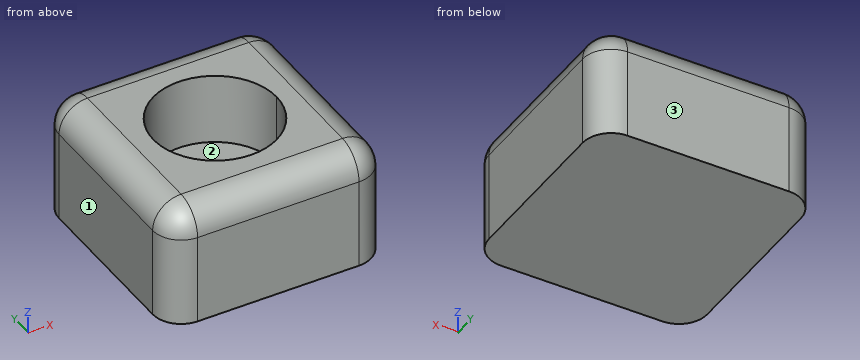
```python
from build123d import *

# Parameters (mm, degrees)
F0_W         = 46
F0_H         = 46
F1_DEPTH     = 25
F3_DEPTH     = 15
F4_R         = 6
F5_T1_DEPTH  = 34
F5_S5_W      = 6
F5_S5_H      = 6
F5_T6_DEPTH  = 6
F5_S11_W     = 6
F5_S11_H     = 6
F5_T12_DEPTH = 6
F5_S17_W     = 6
F5_S17_H     = 6
F5_T18_DEPTH = 6
F5_S23_W     = 6
F5_S23_H     = 6
F5_T24_DEPTH = 6


# Not quite as in the source:
# - a fillet or chamfer that OpenCascade refuses, or shapes differently, is made with other operations: its cross-section is extruded or revolved along the edge and cut away or added


with BuildPart() as f1:
    # F0 (on Top) → F1 (new body)
    with BuildSketch(Plane.XY):
        with Locations((-23, 23)):
            Rectangle(F0_W, F0_H)
    extrude(amount=F1_DEPTH)

    # F2 (on face) → F3 (cut)
    with BuildSketch(Plane.XY.offset(25)):
        with BuildLine():
            ThreePointArc((-10, 23), (-32.1923881554, 32.1923881554), (-23, 10))
            ThreePointArc((-23, 10), (-13.8076118446, 13.8076118446), (-10, 23))
        make_face()
    extrude(amount=-F3_DEPTH, mode=Mode.SUBTRACT)

    # F4
    f4_edges = [f1.edges().sort_by_distance(p)[0] for p in [
        (-23, 0, 25),
        (-46, 23, 25),
        (0, 23, 25),
        (-23, 46, 25),
    ]]
    fillet(f4_edges, radius=F4_R)

    # F5: fillet of radius 6 on 4 edges, made by hand

    # F5_s2 → F5_t1 (cut)
    with BuildSketch(Plane.XY.offset(-15)):
        with BuildLine():
            ThreePointArc((-40, 0), (-44.2426406871, 1.7573593129), (-46, 6))
            Line((-46, 6), (-46, 0))
            Line((-46, 0), (-40, 0))
        make_face()
        with BuildLine():
            ThreePointArc((-6, 0), (-1.7573593129, 1.7573593129), (0, 6))
            Line((0, 6), (0, 0))
            Line((0, 0), (-6, 0))
        make_face()
        with BuildLine():
            ThreePointArc((0, 40), (-1.7573593129, 44.2426406871), (-6, 46))
            Line((-6, 46), (0, 46))
            Line((0, 46), (0, 40))
        make_face()
        with BuildLine():
            ThreePointArc((-46, 40), (-44.2426406871, 44.2426406871), (-40, 46))
            Line((-40, 46), (-46, 46))
            Line((-46, 46), (-46, 40))
        make_face()
    extrude(amount=F5_T1_DEPTH, mode=Mode.SUBTRACT)


with BuildPart() as f5_tool4:
    # F5_s5 → F5_t6 (new body)
    with BuildSketch(Plane.YZ.offset(-40)):
        with Locations((43, 22)):
            Rectangle(F5_S5_W, F5_S5_H)
    extrude(amount=-F5_T6_DEPTH)

    # F5_s7 → F5_t8 (revolve, cut)
    with BuildSketch(Plane(origin=(-40, 40, 19), x_dir=(0, -0.7071067812, -0.7071067812), z_dir=(0, 0.7071067812, -0.7071067812))):
        with BuildLine():
            ThreePointArc((0, -6), (6, 0), (0, 6))
            Line((0, 6), (0, -6))
        make_face()
    revolve(axis=Axis((-40, 40, 19), (-1, 0, 0)), mode=Mode.SUBTRACT)


with BuildPart() as f1_1:
    add(f1.part)

    # F5_t3: cut F5_tool4
    add(f5_tool4.part, mode=Mode.SUBTRACT)


with BuildPart() as f5_tool10:
    # F5_s11 → F5_t12 (new body)
    with BuildSketch(Plane.YZ.offset(-6)):
        with Locations((43, 22)):
            Rectangle(F5_S11_W, F5_S11_H)
    extrude(amount=F5_T12_DEPTH)

    # F5_s13 → F5_t14 (revolve, cut)
    with BuildSketch(Plane(origin=(-6, 40, 19), x_dir=(0, -0.7071067812, -0.7071067812), z_dir=(0, -0.7071067812, 0.7071067812))):
        with BuildLine():
            ThreePointArc((0, -6), (6, 0), (0, 6))
            Line((0, 6), (0, -6))
        make_face()
    revolve(axis=Axis((-6, 40, 19), (1, 0, 0)), mode=Mode.SUBTRACT)


with BuildPart() as f1_2:
    add(f1_1.part)

    # F5_t9: cut F5_tool10
    add(f5_tool10.part, mode=Mode.SUBTRACT)


with BuildPart() as f5_tool16:
    # F5_s17 → F5_t18 (new body)
    with BuildSketch(Plane.XZ.offset(-6)):
        with Locations((-3, 22)):
            Rectangle(F5_S17_W, F5_S17_H)
    extrude(amount=F5_T18_DEPTH)

    # F5_s19 → F5_t20 (revolve, cut)
    with BuildSketch(Plane(origin=(-6, 6, 19), x_dir=(-0.7071067812, 0, -0.7071067812), z_dir=(-0.7071067812, 0, 0.7071067812))):
        with BuildLine():
            ThreePointArc((0, -6), (6, 0), (0, 6))
            Line((0, 6), (0, -6))
        make_face()
    revolve(axis=Axis((-6, 6, 19), (0, -1, 0)), mode=Mode.SUBTRACT)


with BuildPart() as f1_3:
    add(f1_2.part)

    # F5_t15: cut F5_tool16
    add(f5_tool16.part, mode=Mode.SUBTRACT)


with BuildPart() as f5_tool22:
    # F5_s23 → F5_t24 (new body)
    with BuildSketch(Plane.XZ.offset(-6)):
        with Locations((-43, 22)):
            Rectangle(F5_S23_W, F5_S23_H)
    extrude(amount=F5_T24_DEPTH)

    # F5_s25 → F5_t26 (revolve, cut)
    with BuildSketch(Plane(origin=(-40, 6, 19), x_dir=(0.7071067812, 0, -0.7071067812), z_dir=(-0.7071067812, 0, -0.7071067812))):
        with BuildLine():
            ThreePointArc((0, -6), (6, 0), (0, 6))
            Line((0, 6), (0, -6))
        make_face()
    revolve(axis=Axis((-40, 6, 19), (0, -1, 0)), mode=Mode.SUBTRACT)


with BuildPart() as f1_4:
    add(f1_3.part)

    # F5_t21: cut F5_tool22
    add(f5_tool22.part, mode=Mode.SUBTRACT)


solid = f1_4.part
```
For this review, take the finished solid that the model builds, in its own axes (mm). Face numbers are marked on the shaded views. Coordinates: 2 decimals unless noted, no trailing zeros. Loops run counter-clockwise (first coordinate to the right, second up) from the corner with the lowest first, then second, coordinate; pieces in that order, holes last. Notation, with made-up numbers: (-36, -37.75) -> (-3, -37.75) arc R28 ccw to (-3, -3.75) -> close; hole circle Ø8 at (-25, 73). An arc over 180 degrees is marked (long way). Return JSON: item names as keys, results as strings. Group by question number.
(1) To check wall thickness, follow L1, parallel to X at y = 23, z = 13.75; L2, parallel to Y at x = -23, z = 19; L3, parallel to Y at x = -16, z = 19. State the ranges of each line that lie inside material, in increasing order.
(2) Consider section B-B, the plane y = 27. Give the boundary of the cut face in (x, z), plus the area to 3 significant figures.
(3) Consider section D-D, the plane y = 42.5. Give the boundary of the cut face in (x, z).
(4) Consider section A-A, the plane z = 14.25. Give the boundary of the cut face in (x, y), plus the area to 3 significant figures.
(5) Consider section C-C, the plane x = -4.5. Give the boundary of the cut face in (y, z), plus the area to 3 significant figures.
(6) Mouldability with a two-part tool opening along X and no side actions: class the marked faces 1, 2 and 3 as pulls with the +X half, pulls with the -X half, needs draft (parallel to the pull), parting line crosses it, or undercut.
(7) For pin 1 Ø21 at (x, y) = (-23, 23) entering from +Z, flat-tipped, find the tip position at first contact; note if it passes through.
Results below:
{
 "1": {"L1": "x = -46 to -36, -10 to 0", "L2": "y = 0 to 10, 36 to 46", "L3": "y = 0 to 12.05, 33.95 to 46"},
 "2": {"outline": "(-46, 0) -> (0, 0) -> (0, 19) arc R6 ccw to (-6, 25) -> (-10.63, 25) -> (-10.63, 10) -> (-35.37, 10) -> (-35.37, 25) -> (-40, 25) arc R6 ccw to (-46, 19) -> close", "area": "763 mm2"},
 "3": {"outline": "(-45.45, 0) -> (-0.55, 0) -> (-0.55, 19) arc R5.45 ccw to (-6, 24.45) -> (-40, 24.45) arc R5.45 ccw to (-45.45, 19) -> close"},
 "4": {"outline": "(-46, 6) arc R6 ccw to (-40, 0) -> (-6, 0) arc R6 ccw to (0, 6) -> (0, 40) arc R6 ccw to (-6, 46) -> (-40, 46) arc R6 ccw to (-46, 40) -> close; hole circle Ø26 at (-23, 23)", "area": "1,550 mm2"},
 "5": {"outline": "(0.19, 0) -> (45.81, 0) -> (45.81, 19) arc R5.81 ccw to (40, 24.81) -> (6, 24.81) arc R5.81 ccw to (0.19, 19) -> close", "area": "1,120 mm2"},
 "6": {"face 1": "pulls with the -X half", "face 2": "undercut", "face 3": "needs draft"},
 "7": {"pin 1": "stops at z = 10"}
}
